Work out the finished part from the listing and answer in its coordinate system (mm). A direction names the side the tool comes from. Give positions to 0.01 mm unless a question says otherwise; leave off trailing zeros. Order: outer loops, then holes, each group sorted by start corner. A loop starts at its lowest first (then second) coordinate and runs counter-clockwise, first axis right, second up. Notation, with made-up numbers: (24.5, -7.5) -> (46.5, -7.5) arc R19 cw to (46.5, -3.5) -> close; hole circle Ø2 at (-27, -2). An arc over 180 degrees is marked (long way). Answer as CSV lines item,"result". Start each with the question number.
1. For faces 1 (the cylindrical face through (-187.574, 220.113, 1.61)), 2 (the flat face through (-176, 206.019, 2)), determine the directions among +Z, -Z, +X, -X, +Y, -Y from which every point of the face is accessible in a straight line to the end or side of a thin tool.
2. Find the intervals of material crossed by L1, parallel to X at y = 133, z = 2.95; L2, parallel to Y at x = -177.5, z = 1.85; L3, parallel to Y at x = -176, z = 0.4, in increasing order.
3. A cutting plane is placed at B-B (y = 124). Give the vertices of the cut face in (x, z) (3 decimals), then the cut area to 3 significant figures.
4. Flat-ended cylindrical pins translate along their axes: pin 1 (6 mm diameter, centred on x = -143.69, y = 122.99, fed in from +Z); pin 2 (1 mm diameter, centred on x = -180, z = 1.5, fed in from -Y). Find the tip coordinate at first contact, or state that the pin passes through.
5. A cutting plane is placed at D-D (x = -169). Give the vertices of the cut face in (y, z) (3 decimals), then the cut area to 3 significant figures.
6. For a pull along Y with two mould halves and no side action, classify faces 3 (the flat face through (-158.223, 199.115, 1.565)), 4 (the flat face through (-151, 176, 3.175)), 5 (the flat face through (-173, 221.019, 2)), 6 (the cylindrical face through (-146.736, 121.722, 1.565)) as released by +Y, released by -Y, zero draft, split by the parting line, or undercut.
7. A cutting plane is placed at A-A (x = -179). Give the vertices of the cut face in (y, z) (3 decimals).
8. A cutting plane is placed at C-C (z = 0.75). Give the vertices of the cut face in (x, y) (3 decimals), then the cut area to 3 significant figures.
from build123d import *

# Parameters (mm, degrees)
BOSS_EXTRUDE1_DEPTH  = 3.175
M6_CLEARANCE_HOLE1_D = 6.6
FILLET1_R            = 3.175
M8_CLEARANCE_HOLE1_D = 9


with BuildPart() as part:
    # Sketch2 → Boss-Extrude1 (new body)
    with BuildSketch(Plane.XY):
        Polygon((-136.187872738, 122.986389998), (-136.187872738, 198.242289047), (-158.863157835, 221.01860883), (-179.00393221, 221.01860883), (-188.52893221, 221.01860883), (-188.52893221, 206.01860883), (-179.00393221, 206.01860883), (-151.187872738, 206.01860883), (-151.187872738, 122.986389998), (-151.187872738, 115.366389998), (-136.187872738, 115.366389998), align=None)
        Polygon((-151.187872738, 206.01860883), (-165.095902474, 206.01860883), (-151.187872738, 192.04860883), align=None)
    extrude(amount=BOSS_EXTRUDE1_DEPTH)

    # M6 Clearance Hole1 (through all)
    with Locations(Plane.XY.offset(3.175)):
        with Locations((-143.687872738, 122.986389998)):
            Hole(M6_CLEARANCE_HOLE1_D / 2)

    # Fillet1
    fillet1_edges = [part.edges().sort_by_distance(p)[0] for p in [
        (-188.52893221, 206.01860883, 1.5875),
        (-188.52893221, 221.01860883, 1.5875),
        (-158.863157835, 221.01860883, 1.5875),
        (-136.187872738, 198.242289047, 1.5875),
        (-136.187872738, 115.366389998, 1.5875),
        (-151.187872738, 115.366389998, 1.5875),
        (-151.187872738, 192.04860883, 1.5875),
        (-165.095902474, 206.01860883, 1.5875),
    ]]
    fillet(fillet1_edges, radius=FILLET1_R)

    # M8 Clearance Hole1 (through all)
    with Locations(Plane.XY.offset(3.175)):
        with Locations((-179.00393221, 213.51860883)):
            Hole(M8_CLEARANCE_HOLE1_D / 2)


solid = part.part
Answer sheet:
1,face 1,"+Z, -Z, -X, +Y"
1,face 2,"+Z, -Z, -X, -Y"
2,L1,"x = -151.19 to -136.19"
2,L2,"y = 206.02 to 209.28, 217.76 to 221.02"
2,L3,"y = 206.02 to 210.17, 216.87 to 221.02"
3,outline,"(-151.188, 0) -> (-146.828, 0) -> (-146.828, 3.175) -> (-151.188, 3.175) -> close; (-140.547, 0) -> (-136.188, 0) -> (-136.188, 3.175) -> (-140.547, 3.175) -> close"
3,area,"27.7 mm^2"
4,pin 1,"passes through"
4,pin 2,"stops at y = 206.02"
5,outline,"(206.019, 0) -> (221.019, 0) -> (221.019, 3.175) -> (206.019, 3.175) -> close"
5,area,"47.6 mm^2"
6,face 3,"released by -Y"
6,face 4,"zero draft"
6,face 5,"released by +Y"
6,face 6,"undercut"
7,outline,"(206.019, 0) -> (209.019, 0) -> (209.019, 3.175) -> (206.019, 3.175) -> close; (218.019, 0) -> (221.019, 0) -> (221.019, 3.175) -> (218.019, 3.175) -> close"
8,outline,"(-188.529, 209.194) arc R3.175 ccw to (-185.354, 206.019) -> (-166.415, 206.019) arc R3.175 cw to (-164.165, 205.084) -> (-152.113, 192.978) arc R3.175 cw to (-151.188, 190.738) -> (-151.188, 118.541) arc R3.175 ccw to (-148.013, 115.366) -> (-139.363, 115.366) arc R3.175 ccw to (-136.188, 118.541) -> (-136.188, 196.931) arc R3.175 ccw to (-137.113, 199.171) -> (-157.932, 220.084) arc R3.175 ccw to (-160.182, 221.019) -> (-185.354, 221.019) arc R3.175 ccw to (-188.529, 217.844) -> close; hole circle Ø9 at (-179.004, 213.519); hole circle Ø6.6 at (-143.688, 122.986)"
8,area,"1,880 mm^2"
